Work out the finished part from the listing and answer in its coordinate system (mm). A direction names the side the tool comes from. Coordinates: 2 decimals unless noted, no trailing zeros. Order: outer loops, then holes, each group sorted by start corner. A loop starts at its lowest first (then second) coordinate and runs counter-clockwise, first axis right, second up. Notation, with made-up numbers: M -39,84 L -10,84 A24 ccw -10,100 Z; hole C 58.5,-31 d3. An arc over 180 degrees is marked long. Use a Markdown table: item, result.
from build123d import *

# Parameters (mm, degrees)
BOSS_EXTRU_1_DEPTH      = 120
COQUE1_START            = 10
COQUE1_DEPTH            = 100
ESQUISSE3_W             = 75
ESQUISSE3_H             = 75
ENL_V_MAT_EXTRU_1_DEPTH = 5
ENL_V_MAT_EXTRU_2_REACH = 194.855
ESQUISSE4_W             = 30
ESQUISSE4_H             = 30
ESQUISSE5_R             = 3.25
ENL_V_MAT_EXTRU_3_DEPTH = 3.5
ENL_V_START             = 50
ESQUISSE6_R             = 3.75
ENL_V_MAT_EXTRU_4_DEPTH = 10
ESQUISSE7_W             = 14
ESQUISSE7_H             = 12
ENL_V_MAT_EXTRU_5_DEPTH = 8
ESQUISSE8_W             = 37.840944821
ESQUISSE8_H             = 24.41449918
ENL_V_MAT_EXTRU_6_DEPTH = 10
ENL_V_START_2           = 145.39392
ESQUISSE9_R             = 3.5
ENL_V_MAT_EXTRU_8_DEPTH = 25


# Read off the part's stored shape, not the designer's step: Coque1
with BuildPart() as part:
    # Esquisse1 → Boss.-Extru.1 (new body)
    with BuildSketch(Plane(origin=(0, 0, 0), x_dir=(0, 0, -1), z_dir=(1, 0, 0))):
        with BuildLine():
            Line((0, 0), (-100, 0))
            Line((-100, 0), (-100, 50))
            ThreePointArc((-100, 50), (-97.071067812, 57.071067812), (-90, 60))
            Line((-90, 60), (-67.337993857, 60))
            ThreePointArc((-67.337993857, 60), (-61.421914074, 61.937742252), (-57.798601843, 67))
            Line((-57.798601843, 67), (-30, 155.393920142))
            Line((-30, 155.393920142), (0, 155.393920142))
            Line((0, 155.393920142), (0, 0))
        make_face()
    extrude(amount=BOSS_EXTRU_1_DEPTH)

    # Coque1 outline → Coque1 (cut)
    with BuildSketch(Plane.YZ.offset(COQUE1_START)):
        with BuildLine():
            Line((145.393920142, 0), (145.393920142, 22.662006143))
            Line((145.393920142, 22.662006143), (64, 48.259209829))
            ThreePointArc((64, 48.259209829), (53.875484503, 55.505834291), (50, 67.337993857))
            Line((50, 67.337993857), (50, 90))
            Line((50, 90), (10, 90))
            Line((10, 90), (10, 0))
            Line((10, 0), (145.393920142, 0))
        make_face()
    extrude(amount=COQUE1_DEPTH, mode=Mode.SUBTRACT)

    # Esquisse3 → Enlèv. mat.-Extru.1 (cut)
    with BuildSketch(Plane(origin=(0, 22.570905626, 71.770905626), x_dir=(-1, 0, 0), z_dir=(0, -0.3000000000000002, -0.9539392014169457))):
        with Locations((-60, 92.905349014)):
            Rectangle(ESQUISSE3_W, ESQUISSE3_H)
    extrude(amount=ENL_V_MAT_EXTRU_1_DEPTH, mode=Mode.SUBTRACT)

    # Esquisse4 → Enlèv. mat.-Extru.2 (cut, up to next)
    with BuildSketch(Plane(origin=(0, 22.570905626, 71.770905626), x_dir=(-1, 0, 0), z_dir=(0, -0.3000000000000002, -0.9539392014169457)), mode=Mode.PRIVATE) as enl_v_mat_extru_2_sk1:
        with Locations((-37.5, 115.405349014)):
            Rectangle(ESQUISSE4_W, ESQUISSE4_H)
    enl_v_mat_extru_2_tool1 = extrude(enl_v_mat_extru_2_sk1.sketch, amount=ENL_V_MAT_EXTRU_2_REACH, mode=Mode.PRIVATE) & part.part
    # Esquisse4 → Enlèv. mat.-Extru.2 (cut, up to next)
    with BuildSketch(Plane(origin=(0, 22.570905626, 71.770905626), x_dir=(-1, 0, 0), z_dir=(0, -0.3000000000000002, -0.9539392014169457)), mode=Mode.PRIVATE) as enl_v_mat_extru_2_sk2:
        with Locations((-37.5, 70.405349014)):
            Rectangle(ESQUISSE4_W, ESQUISSE4_H)
    enl_v_mat_extru_2_tool2 = extrude(enl_v_mat_extru_2_sk2.sketch, amount=ENL_V_MAT_EXTRU_2_REACH, mode=Mode.PRIVATE) & part.part
    # Esquisse4 → Enlèv. mat.-Extru.2 (cut, up to next)
    with BuildSketch(Plane(origin=(0, 22.570905626, 71.770905626), x_dir=(-1, 0, 0), z_dir=(0, -0.3000000000000002, -0.9539392014169457)), mode=Mode.PRIVATE) as enl_v_mat_extru_2_sk3:
        with Locations((-82.5, 115.405349014)):
            Rectangle(ESQUISSE4_W, ESQUISSE4_H)
    enl_v_mat_extru_2_tool3 = extrude(enl_v_mat_extru_2_sk3.sketch, amount=ENL_V_MAT_EXTRU_2_REACH, mode=Mode.PRIVATE) & part.part
    # Esquisse4 → Enlèv. mat.-Extru.2 (cut, up to next)
    with BuildSketch(Plane(origin=(0, 22.570905626, 71.770905626), x_dir=(-1, 0, 0), z_dir=(0, -0.3000000000000002, -0.9539392014169457)), mode=Mode.PRIVATE) as enl_v_mat_extru_2_sk4:
        with Locations((-82.5, 70.405349014)):
            Rectangle(ESQUISSE4_W, ESQUISSE4_H)
    enl_v_mat_extru_2_tool4 = extrude(enl_v_mat_extru_2_sk4.sketch, amount=ENL_V_MAT_EXTRU_2_REACH, mode=Mode.PRIVATE) & part.part
    add(enl_v_mat_extru_2_tool1.solids().sort_by_distance((37.5, 132.660592, 37.149301))[0], mode=Mode.SUBTRACT)
    add(enl_v_mat_extru_2_tool2.solids().sort_by_distance((37.5, 89.733328, 50.649301))[0], mode=Mode.SUBTRACT)
    add(enl_v_mat_extru_2_tool3.solids().sort_by_distance((82.5, 132.660592, 37.149301))[0], mode=Mode.SUBTRACT)
    add(enl_v_mat_extru_2_tool4.solids().sort_by_distance((82.5, 89.733328, 50.649301))[0], mode=Mode.SUBTRACT)

    # Esquisse5 → Enlèv. mat.-Extru.3 (cut)
    with BuildSketch(Plane(origin=(0, 0, 0), x_dir=(-1, 0, 0), z_dir=(0, 0, -1))):
        with Locations(Location((-114.715748307, 149.926194797, 0), (0, 0, 90))):
            Circle(ESQUISSE5_R)
        with Locations(Location((-5.284251693, 149.926194797, 0), (0, 0, 270))):
            Circle(ESQUISSE5_R)
        with Locations(Location((-5.284251693, 5.467725345, 0), (0, 0, 90))):
            Circle(ESQUISSE5_R)
        with Locations(Location((-114.715748307, 5.467725345, 0), (0, 0, 270))):
            Circle(ESQUISSE5_R)
    extrude(amount=-ENL_V_MAT_EXTRU_3_DEPTH, mode=Mode.SUBTRACT)

    # Esquisse6 → Enlèv. mat.-Extru.4 (cut)
    with BuildSketch(Plane(origin=(0, 0, 0), x_dir=(1, 0, 0), z_dir=(0, 1, 0)).offset(ENL_V_START)):
        with Locations(Location((60, -80, 0), (0, 0, 90))):
            Circle(ESQUISSE6_R)
    extrude(amount=ENL_V_MAT_EXTRU_4_DEPTH, mode=Mode.SUBTRACT)

    # Esquisse7 → Enlèv. mat.-Extru.5 (cut)
    with BuildSketch(Plane(origin=(0, 0, 0), x_dir=(1, 0, 0), z_dir=(0, 1, 0)).offset(ENL_V_START)):
        with Locations((60, -80)):
            Rectangle(ESQUISSE7_W, ESQUISSE7_H)
    extrude(amount=ENL_V_MAT_EXTRU_5_DEPTH, mode=Mode.SUBTRACT)

    # Esquisse8 → Enlèv. mat.-Extru.6 (cut)
    with BuildSketch(Plane(origin=(120, 0, 0), x_dir=(0, 0, -1), z_dir=(1, 0, 0))):
        with Locations((-18.920472411, 24.304309827)):
            Rectangle(ESQUISSE8_W, ESQUISSE8_H)
    extrude(amount=-ENL_V_MAT_EXTRU_6_DEPTH, mode=Mode.SUBTRACT)

    # Esquisse9 → Enlèv. mat.-Extru.8 (cut)
    with BuildSketch(Plane(origin=(0, 0, 0), x_dir=(1, 0, 0), z_dir=(0, 1, 0)).offset(ENL_V_START_2)):
        with Locations((60, 0)):
            Circle(ESQUISSE9_R)
    extrude(amount=ENL_V_MAT_EXTRU_8_DEPTH, mode=Mode.SUBTRACT)


solid = part.part
(1) A cutting plane is placed at B-B (y = 33.5). Determine the outline of the cut face in (x, z), then the cut area to 3 significant figures.
Conclusion:
| item | result |
|---|---|
| outline | M 0,0 L 10,0 L 10,90 L 110,90 L 110,37.84 L 120,37.84 L 120,100 L 0,100 Z |
| area | 2,620 mm2 |
(2) A cutting plane is placed at C-C (z = 71). Determine the outline of the cut face in (x, y), then the cut area to 3 significant figures.
Conclusion:
| item | result |
|---|---|
| outline | M 0,0 L 120,0 L 120,60 L 0,60 Z; hole M 10,10 L 110,10 L 110,50 L 10,50 Z |
| area | 3,200 mm2 |
(3) Determine the mould class of faces 5 (the flat face through (59, 0, 49)), 6 (the cylindrical face through (4.308, 146.826, 1.726)), 7 (the flat face through (60, 58, 76)), 8 (the cylindrical face through (59.16, 61.89, 61.49)) for opening direction Y: pulls with the +Y half, pulls with the -Y half, needs draft (parallel to the pull), parting line crosses it, or undercut.
Conclusion:
| item | result |
|---|---|
| face 5 | pulls with the -Y half |
| face 6 | undercut |
| face 7 | undercut |
| face 8 | pulls with the +Y half |
(4) A cutting plane is placed at D-D (x = 33). Determine the outline of the cut face in (y, z).
Conclusion:
| item | result |
|---|---|
| outline | M 0,0 L 10,0 L 10,90 L 50,90 L 50,67.34 A20 ccw 64,48.26 L 72.42,45.61 L 75.42,55.15 L 67,57.8 A10 cw 60,67.34 L 60,90 A10 ccw 50,100 L 0,100 Z; M 101.04,36.61 L 115.35,32.11 L 116.85,36.88 L 102.54,41.38 Z; M 143.97,23.11 L 145.39,22.66 L 145.39,0 L 155.39,0 L 155.39,30 L 146.97,32.65 Z |
(5) Given P1, Ø6, axis at y = 90.5, z = 38, coming from the -X side; P2, Ø25, axis at x = 71, z = 78, coming from the +Y side; P3, Ø8, axis at x = 56, y = 137.5, coming from the -Z side; P4, Ø2, axis at x = 115, y = 4.5, coming from the -Z side, each flat-ended and moving along its own axis, determine where each tip first touches the part or whether it passes through.
Conclusion:
| item | result |
|---|---|
| P1 | x = 0 |
| P2 | y = 60.17 |
| P3 | z = 23.89 |
| P4 | z = 3.5 |
(6) Straight lines are drawn through the part: L1, parallel to X at y = 56.5, z = 49; L2, parallel to Y at x = 101, z = 75.5; L3, parallel to X at y = 125, z = 34.5. For each, find the intervals that lie inside material, in ascending order.
Conclusion:
| item | result |
|---|---|
| L1 | 0 to 10, 110 to 120 |
| L2 | 0 to 10, 50 to 60 |
| L3 | 0 to 22.5, 97.5 to 120 |
(7) Which of the six approach directions +Z, -Z, +X, -X, +Y, -Y give full straight-line access (tool end or side, diameter ignored) to faces 1 (the cylindrical face through (61.436, 58.986, 76.536)), 2 (the flat face through (67, 54, 80)), 3 (the cylindrical face through (59.3, 53.981, 55.363)), 4 (the flat face through (60.525, 145.824, 29.006))?
Conclusion:
| item | result |
|---|---|
| face 1 | +Y |
| face 2 | none |
| face 3 | -Z |
| face 4 | +Z |
(8) A cutting plane is placed at A-A (x = 60). Determine the outline of the cut face in (y, z), then the cut area to 3 significant figures.
Conclusion:
| item | result |
|---|---|
| outline | M 0,0 L 10,0 L 10,90 L 50,90 L 50,86 L 58,86 L 58,83.75 L 60,83.75 L 60,90 A10 ccw 50,100 L 0,100 Z; M 50,67.34 A20 ccw 64,48.26 L 145.39,22.66 L 145.39,3.5 L 155.39,3.5 L 155.39,30 L 146.97,32.65 L 145.47,27.88 L 73.92,50.38 L 75.42,55.15 L 67,57.8 A10 cw 60,67.34 L 60,76.25 L 58,76.25 L 58,74 L 50,74 Z |
| area | 2,530 mm2 |
